Work out the finished part from the listing and answer in its coordinate system (mm). Face numbers are marked on the shaded views. A direction names the side the tool comes from. Coordinates: 2 decimals unless noted, no trailing zeros. Order: outer loops, then holes, each group sorted by start corner. A loop starts at its lowest first (then second) coordinate and runs counter-clockwise, first axis right, second up. Notation, with made-up numbers: M -31,57.5 L 28,57.5 A9 ccw 28,65.5 Z; hole C -33,-6.75 d5. An arc over 180 degrees is marked long. Write item = value, one per line. Start each with the question number.
Q1. Straight lines are drawn through the part: line 1 along Y through (x, z) = (-1.5, 25.5); line 2 along Z through (x, y) = (-12, -64); line 3 along X through (y, z) = (67.5, 8). For each, find the intervals that lie inside material, in ascending order.
Q2. Find section B-B on y = -12.5. Give the vertices of the cut face in (x, z), and give its area (3 significant figures).
Q3. Find section A-A on z = 8.5. Give the vertices of the cut face in (x, y), and give its area (3 significant figures).
Q4. Each of these flat-tipped pins is pushed along its axis until it touches: P1, Ø12, axis at x = -32, y = -94.5, coming from the +Z side; P2, Ø1.5, axis at x = -22, z = 6, coming from the +Y side; P3, Ø1.5, axis at x = -32.5, y = 125, coming from the -Z side; P4, Ø2, axis at x = -23.5, z = 3, coming from the -Y side. Where does it stop, or does it pass through?
Q5. A tool of negligible diameter and unlimited length cuts with its end or side. For the marked faces 1 and 2, from which of +Z, -Z, +X, -X, +Y, -Y can it reach the whole face along a straight path? Write none if from no direction.
Q6. Find section C-C on x = -33. Give the vertices of the cut face in (y, z).
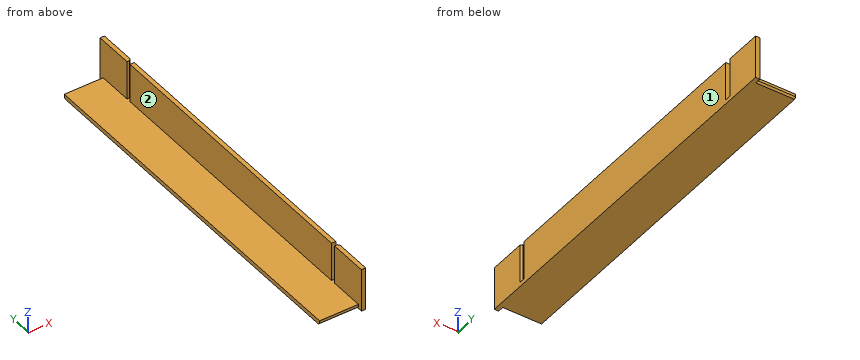
Solid Edge part; units mm, degrees
sketch "Sketch1" plane through (-9.04, 0, 33.0648) normal (0, -1, 0) x (1, 0, 0)
  line L0 (-30.96, -29.0648) -> (5.04, -29.0648)
  line L1 (5.04, -29.0648) -> (5.04, 6.9352)
  line L2 (5.04, 6.9352) -> (9.04, 6.9352)
  line L3 (9.04, 6.9352) -> (9.04, -33.0648)
  line L4 (9.04, -33.0648) -> (-30.96, -33.0648)
  line L5 (-30.96, -33.0648) -> (-30.96, -29.0648)
extrude "Protrusion1" add sketch "Sketch1" along normal mid plane 350
sketch "Sketch2" plane through (-20, 0, 0) normal (0, 0, -1) x (0, 1, 0)
  line L0 (-175, -20) -> (-171, -20)
  line L1 (-171, -20) -> (-171, 16)
  line L2 (-171, 16) -> (-175, 16)
  line L3 (-175, 16) -> (-175, -20)
  dimension "D1" = 175
extrude "Cutout1" cut sketch "Sketch2" against normal up to next
sketch "Sketch3" plane through (0, 0, 20) normal (1, 0, 0) x (0, 1, 0)
  line L0 (-139, -16) -> (-135, -16)
  line L1 (-135, -16) -> (-135, 20)
  line L2 (-135, 20) -> (-139, 20)
  line L3 (-139, 20) -> (-139, -16)
  dimension "D1" = 135
extrude "Cutout2" cut sketch "Sketch3" against normal up to next
mirror "Mirror1" about plane through (0, 0, 0) normal (0, -1, 0) of "Cutout1", "Cutout2"
chamfer "Fase_3" distance 1.5 angle 45 4 edges at (0, -139, 22) (-22, -171, 0) (-22, 171, 0) (0, 139, 22)
Findings below:
q1.line_1 = -175 to -139, -135 to 135, 139 to 175
q1.line_2 = 0 to 4
q1.line_3 = -4 to 0
q2.outline = M -40,0 L 0,0 L 0,40 L -4,40 L -4,4 L -40,4 Z
q2.area = 304 mm^2
q3.outline = M -4,-175 L 0,-175 L 0,-140.5 L -1.5,-139 L -4,-139 Z; M -4,-135 L 0,-135 L 0,135 L -4,135 Z; M -4,139 L -1.5,139 L 0,140.5 L 0,175 L -4,175 Z
q3.area = 1,370 mm^2
q4.P1 = 4
q4.P2 = through
q4.P3 = 0
q4.P4 = -171
q5.face_1 = +Z, -Z, +X, +Y, -Y
q5.face_2 = +Z, -X, +Y, -Y
q6.outline = M -171,1.5 L -169.5,0 L 169.5,0 L 171,1.5 L 171,4 L -171,4 Z
